```python
from build123d import *
from build123d.topology import SkipClean

# Parameters (mm, degrees)
SKETCH_1_W          = 40
SKETCH_1_H          = 42
SKETCH_1_R          = 1.6
EXTRUDE_1_DEPTH     = 10.5
FILLET_1_R          = 2
SKETCH_2_R          = 1.6
CUT_EXTRUDE_1_DEPTH = 89.183048258
EXTRUDE_START       = -10.5
SKETCH_3_R          = 1.6
EXTRUDE_2_DEPTH     = 10.5
SKETCH_4_R          = 3.5
CUT_EXTRUDE_2_DEPTH = 5
CUT_EXTRUDE_3_DEPTH = 88.728273664
SKETCH_6_W          = 11
SKETCH_6_H          = 11
CUT_EXTRUDE_4_DEPTH = 89.183048258
FILLET_2_R          = 1


with BuildPart() as part:
    # 草图1 → 凸台-拉伸1 (new body)
    with BuildSketch(Plane(origin=(0, 0, 0), x_dir=(1, 0, 0), z_dir=(0, 1, 0))):
        with Locations((-65, 0)):
            Rectangle(SKETCH_1_W, SKETCH_1_H)
        with Locations(Location((-79, -17, 0), (0, 0, 90))):
            Circle(SKETCH_1_R, mode=Mode.SUBTRACT)
        with Locations(Location((-69, 0, 0), (0, 0, 90))):
            Circle(SKETCH_1_R, mode=Mode.SUBTRACT)
        with Locations(Location((-79, 17, 0), (0, 0, 90))):
            Circle(SKETCH_1_R, mode=Mode.SUBTRACT)
    extrude(amount=EXTRUDE_1_DEPTH)

    # 圆角1
    fillet_1_edges = [part.edges().sort_by_distance(p)[0] for p in [
        (-45, 5.25, -21),
        (-45, 5.25, 21),
        (-85, 5.25, 21),
        (-85, 5.25, -21),
    ]]
    fillet(fillet_1_edges, radius=FILLET_1_R)

    # 草图2 → 切除-拉伸1 (cut, through all)
    with BuildSketch(Plane(origin=(0, 10.5, 0), x_dir=(1, 0, 0), z_dir=(0, 1, 0))):
        with Locations(Location((-74, 0, 0), (0, 0, 270))):
            Circle(SKETCH_2_R)
        with Locations((-44, 0)):
            Circle(SKETCH_2_R)
        with Locations(Location((-58.4, 0, 0), (0, 0, 270))):
            Circle(SKETCH_2_R)
    extrude(amount=-CUT_EXTRUDE_1_DEPTH, mode=Mode.SUBTRACT)

    # 草图3 → 凸台-拉伸2 (add)
    with BuildSketch(Plane(origin=(0, 10.5, 0), x_dir=(1, 0, 0), z_dir=(0, 1, 0)).offset(EXTRUDE_START)):
        with Locations((-69, 0)):
            Circle(SKETCH_3_R)
    extrude(amount=EXTRUDE_2_DEPTH)

    # 草图4 → 切除-拉伸2 (cut)
    with BuildSketch(Plane(origin=(0, 10.5, 0), x_dir=(1, 0, 0), z_dir=(0, 1, 0))):
        with Locations(Location((-74, 0, 0), (0, 0, 270))):
            Circle(SKETCH_4_R)
        with Locations(Location((-58.4, 0, 0), (0, 0, 270))):
            Circle(SKETCH_4_R)
        with Locations((-43.663101604, 0)):
            Circle(SKETCH_4_R)
    extrude(amount=-CUT_EXTRUDE_2_DEPTH, mode=Mode.SUBTRACT)

    # 草图5 → 切除-拉伸3 (cut, through all)
    with SkipClean():  # the faces are left unmerged after this step: merging them gives an invalid solid
        with BuildSketch(Plane(origin=(0, 5.5, 0), x_dir=(1, 0, 0), z_dir=(0, 1, 0))):
            with BuildLine():
                Line((-45, 3.234610128), (-45, -3.234610128))
                ThreePointArc((-45, -3.234610128), (-47.163101604, 0), (-45, 3.234610128))
            make_face()
        extrude(amount=-CUT_EXTRUDE_3_DEPTH, mode=Mode.SUBTRACT)

    # 草图6 → 切除-拉伸4 (cut, through all)
    with SkipClean():  # the faces are left unmerged after this step: merging them gives an invalid solid
        with BuildSketch(Plane(origin=(0, 10.5, 0), x_dir=(1, 0, 0), z_dir=(0, 1, 0))):
            with Locations((-68.5, 12.5)):
                Rectangle(SKETCH_6_W, SKETCH_6_H)
            with Locations((-53.5, 12.5)):
                Rectangle(SKETCH_6_W, SKETCH_6_H)
            with Locations((-68.5, -12.5)):
                Rectangle(SKETCH_6_W, SKETCH_6_H)
            with Locations((-53.5, -12.5)):
                Rectangle(SKETCH_6_W, SKETCH_6_H)
        extrude(amount=-CUT_EXTRUDE_4_DEPTH, mode=Mode.SUBTRACT)

    # 圆角2
    fillet_2_edges = [part.edges().sort_by_distance(p)[0] for p in [
        (-59, 5.25, -18),
        (-48, 5.25, -18),
        (-48, 5.25, -7),
        (-59, 5.25, -7),
        (-74, 5.25, 7),
        (-63, 5.25, 7),
        (-63, 5.25, 18),
        (-74, 5.25, 18),
        (-59, 5.25, 7),
        (-48, 5.25, 7),
        (-48, 5.25, 18),
        (-59, 5.25, 18),
        (-63, 5.25, -18),
        (-63, 5.25, -7),
        (-74, 5.25, -7),
        (-74, 5.25, -18),
        (-45, 2.75, -3.234610128),
        (-45, 2.75, 3.234610128),
    ]]
    fillet(fillet_2_edges, radius=FILLET_2_R)


solid = part.part
```
Verification items for the finished model (mm, model axes). A direction names the side the tool comes from. Round coordinates to 2 decimals unless told otherwise and drop trailing zeros. Write each loop counter-clockwise with the first axis right and the second up, starting at its lowest first coordinate (ties: lowest second). Pieces come first, ordered by that corner, then holes. Notation, with made-up numbers: (48.5, -28) - (84.5, -28) arc R29 ccw to (84.5, -3) - close; hole circle Ø6 at (-31.5, 62). An arc over 180 degrees is marked (long way). Answer as a JSON object with one key per item and string values. Group by question number.
Q1. Thickness scan on line 1 (Z direction, x = -50.5, y = 5.5); line 2 (X direction, y = 6.5, z = 14.5); line 3 (X direction, y = 6.5, z = -17). Record the ranges inside material, lowest first.
Q2. Mould release check, pull along X, two halves, no side actions. Record for faces 4 (the flat face through (-85, 5, 0)), 5 (the cylindrical face through (-73.699, 5.176, -17.715)), 6 (the flat face through (-65, 0, 0)): released by +X, released by -X, zero draft, split by the parting line, or undercut.
Q3. Section check A-A, the plane x = -52. Enter the section's corners in (y, z).
Q4. Section check B-B, the plane z = -10.5. Enter the section's corners in (x, y), plus the area to 3 significant figures.
Q5. Section check C-C, the plane y = 6.5. Give the number of separate pieces and of enclosed holes in the cut face, plus the area to 3 significant figures.
Q6. Go/stop test with a flat-tipped pin: pin 1 Ø6.5 at (x, z) = (-74, 0) entering from +Y. Record where the tip stops, or that it passes through.
Q7. Tool access check on faces 1 (the flat face through (-65, 5, -21)), 2 (the cylindrical face through (-77.417, 8.035, -0.759)), 3 (the flat face through (-69, 5, -7)). Record the directions out of +Z, -Z, +X, -X, +Y, -Y that give a thin tool (end or side, any length) a straight path to the whole face; none if there is none.
Found:
{
 "1": {"line 1": "z = -21 to -18, -7 to 7, 18 to 21", "line 2": "x = -85 to -74, -63 to -59, -48 to -45", "line 3": "x = -85 to -80.6, -77.4 to -74, -63 to -59, -48 to -45"},
 "2": {"face 4": "released by -X", "face 5": "undercut", "face 6": "zero draft"},
 "3": {"outline": "(0, -21) - (10.5, -21) - (10.5, -18) - (0, -18) - close; (0, -7) - (10.5, -7) - (10.5, 7) - (0, 7) - close; (0, 18) - (10.5, 18) - (10.5, 21) - (0, 21) - close"},
 "4": {"outline": "(-85, 0) - (-74, 0) - (-74, 10.5) - (-85, 10.5) - close; (-63, 0) - (-59, 0) - (-59, 10.5) - (-63, 10.5) - close; (-48, 0) - (-45, 0) - (-45, 10.5) - (-48, 10.5) - close", "area": "189 mm^2"},
 "5": {"separate pieces": "1", "enclosed holes": "8", "area": "1,090 mm^2"},
 "6": {"pin 1": "stops at y = 5.5"},
 "7": {"face 1": "-Z, +X, -X, +Y, -Y", "face 2": "+Y", "face 3": "+Y, -Y"}
}
